from build123d import *

# Parameters (mm, degrees)
BOSS_EXTRUDE1_DEPTH = 4
BOSS_EXTRUDE2_DEPTH = 5


with BuildPart() as part:
    # Sketch1 → Boss-Extrude1 (new body)
    with BuildSketch(Plane.XY):
        with BuildLine():
            Line((-12.5, 0), (-6.723761618, 19.947056679))
            ThreePointArc((-6.723761618, 19.947056679), (0, 25), (6.723761618, 19.947056679))
            Line((6.723761618, 19.947056679), (12.5, 0))
            Line((12.5, 0), (-12.5, 0))
        make_face()
    extrude(amount=BOSS_EXTRUDE1_DEPTH)

    # Sketch2 → Boss-Extrude2 (add)
    with BuildSketch(Plane.XY.offset(4)):
        Polygon((-12.5, 0), (12.5, 0), (11.341686074, 4), (-11.341686074, 4), align=None)
    extrude(amount=BOSS_EXTRUDE2_DEPTH)


solid = part.part
Can you work these out from the model? Positions are in its coordinate system, mm. A direction names the side the tool comes from. Round coordinates to 2 decimals unless told otherwise and drop trailing zeros. Loops run counter-clockwise (first coordinate to the right, second up) from the corner with the lowest first, then second, coordinate; pieces in that order, holes last. Notation, with made-up numbers: (73.25, 37.5) - (124.25, 37.5) arc R16 cw to (124.25, 56.5) - close; hole circle Ø10 at (19, -28). An arc over 180 degrees is marked (long way). Use CSV: the item, a comma, the result in double quotes. Start each with the question number.
1) For faces 1 (the flat face through (0, 4, 6)), 2 (the flat face through (0, 10, 0)), which set-ups out of +Z, -Z, +X, -X, +Y, -Y let a thin tool reach every point of the face, with its end or its side?
2) If we section it at D-D on x = -6.25: Write out the boundary of the cut face in (y, z), plus the area to 3 significant figures.
3) If we section it at C-C on y = 12: Write out the boundary of the cut face in (x, z), plus the area to 3 significant figures.
4) If we section it at A-A on z = 2.5: Write out the boundary of the cut face in (x, y), plus the area to 3 significant figures.
5) If we section it at B-B on x = 0.25: Write out the boundary of the cut face in (y, z), plus the area to 3 significant figures.
6) Please list where these lines run through material, in increasing order: probe 1 along Z at (x, y) = (-0.5, 20); probe 2 along X at (y, z) = (17.25, 3). Write a range as [from, to].
7) For pin 1 Ø6.5 at (x, y) = (3.5, 15) entering from +Z; pin 2 Ø4 at (x, y) = (-9.5, 5) entering from -Z; pin 3 Ø5 at (y, z) = (19, 4) entering from -X; pin 4 Ø5 at (x, z) = (8.5, 2) entering from +Y, each with a flat end and sliding along its axis, tell me the tip position at first contact or that it passes through.
Geometry results:
1,face 1,"+Z, +X, -X, +Y"
1,face 2,"-Z, +X, -X, +Y, -Y"
2,outline,"(0, 0) - (21.15, 0) - (21.15, 4) - (4, 4) - (4, 9) - (0, 9) - close"
2,area,"105 mm2"
3,outline,"(-9.03, 0) - (9.03, 0) - (9.03, 4) - (-9.03, 4) - close"
3,area,"72.2 mm2"
4,outline,"(-12.5, 0) - (12.5, 0) - (6.72, 19.95) arc R7 ccw to (-6.72, 19.95) - close"
4,area,"434 mm2"
5,outline,"(0, 0) - (25, 0) - (25, 4) - (4, 4) - (4, 9) - (0, 9) - close"
5,area,"120 mm2"
6,probe 1,"z = [0, 4]"
6,probe 2,"x = [-7.5, 7.5]"
7,pin 1,"stops at z = 4"
7,pin 2,"stops at z = 0"
7,pin 3,"stops at x = -7.72"
7,pin 4,"stops at y = 21.61"
